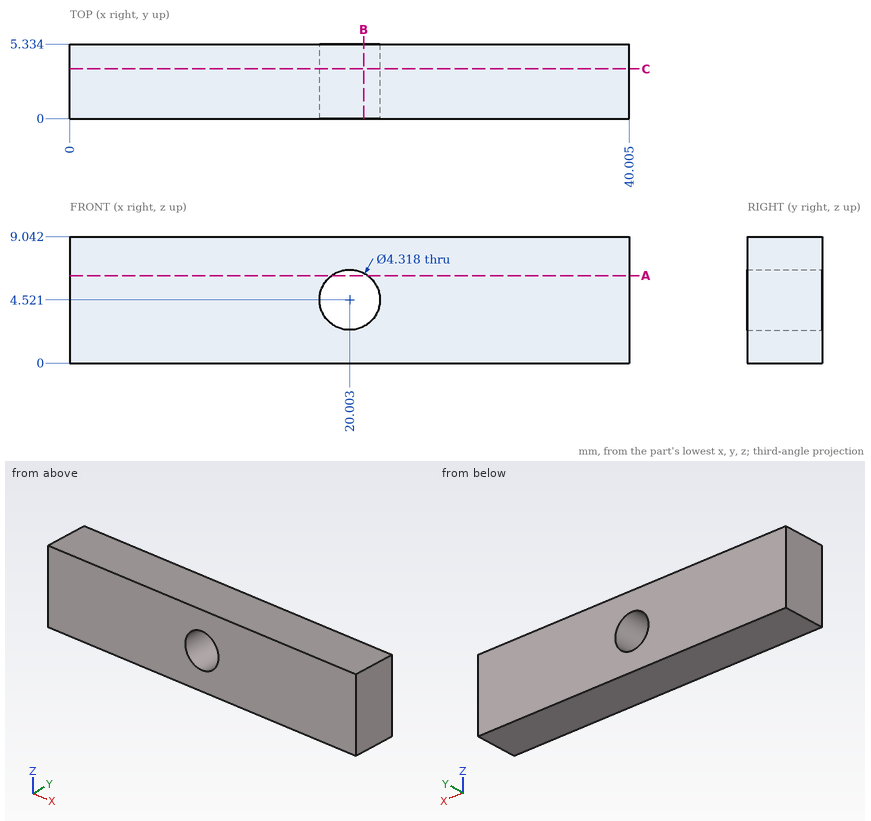
Here's the drawing with two shaded views (mm, measured from the low corner). I have some questions. Give positions to 0.01 mm unless a question says otherwise; leave off trailing zeros. Write each loop counter-clockwise with the first axis right and the second up, starting at its lowest first coordinate (ties: lowest second). Pieces come first, ordered by that corner, then holes. Notation, with made-up numbers: (-30.75, -12.75) - (-24.75, -12.75) arc R9 ccw to (-24.75, 3.25) - close; hole circle Ø10 at (-21, 18.5). An arc over 180 degrees is marked (long way). One line per item, written item: value. Start each with the question number.
Item 1: I'm going to push a flat-ended pin straight in: pin 1 (4 mm diameter, centred on x = 20, z = 4.52, fed in from -Y). Where does the tip first touch, or does it pass through?
Item 2: Please list where these lines run through material, in increasing order: line 1 (X direction, y = 3.1, z = 3.75) (1 decimal); line 2 (X direction, y = 0.7, z = 3.5) (1 decimal); line 3 (Z direction, x = 21, y = 2.05) (1 decimal). Write a range as from..to.
Item 3: Imagine slicing it at A-A, the plane z = 6.25. List the corners of the cut face in (x, y) for me (1 decimal).
Item 4: Imagine slicing it at C-C, the plane y = 3.55. List the corners of the cut face in (x, z) for me (1 decimal), and give its area (3 significant figures).
Item 5: Imagine slicing it at B-B, the plane x = 21. List the corners of the cut face in (y, z) for me (1 decimal).
Geometry says:
1. pin 1: through
2. line 1: 0..18, 22..40
2. line 2: 0..18.1, 21.9..40
2. line 3: 0..2.6, 6.4..9
3. outline: (0, 0) - (18.7, 0) - (18.7, 5.3) - (0, 5.3) - close; (21.3, 0) - (40, 0) - (40, 5.3) - (21.3, 5.3) - close
4. outline: (0, 0) - (40, 0) - (40, 9) - (0, 9) - close; hole circle Ø4.3 at (20, 4.5)
4. area: 347 mm^2
5. outline: (0, 0) - (5.3, 0) - (5.3, 2.6) - (0, 2.6) - close; (0, 6.4) - (5.3, 6.4) - (5.3, 9) - (0, 9) - close
